Check sheet for the drawn part. Datum: minimum x, y, z corner. Units: mm. Give positions to 0.01 mm unless a question says otherwise; leave off trailing zeros. Write each loop counter-clockwise with the first axis right and the second up, starting at its lowest first coordinate (ties: lowest second). Pieces come first, ordered by that corner, then holes. Notation, with made-up numbers: (80, 10.25) -> (111, 10.25) arc R22 cw to (111, 40.25) -> close; hole circle Ø10 at (3.25, 41.25). An arc over 180 degrees is marked (long way). Write item = value, one per line. Start each with the question number.
1. Depth check by flat-ended pin: P1, Ø1.5, axis at x = 30, z = 3, coming from the -Y side; P2, Ø2, axis at y = 32.5, z = 3, coming from the +X side; P3, Ø0.7, axis at x = 29.5, z = 3, coming from the +Y side; P4, Ø5, axis at x = 24, y = 18.5, coming from the -Z side. Enter the tip coordinate at first touch or a pass-through.
2. Cross-section at D-D, the plane x = 26. Record the cut outline in (y, z).
3. Thickness scan on line 1 along Y through (x, z) = (16, 3.2); line 2 along Z through (x, y) = (30, 46); line 3 along X through (y, z) = (10, 5). Record the ranges inside material, lowest first.
4. Cross-section at A-A, the plane x = 16. Record the cut outline in (y, z).
5. Cross-section at B-B, the plane y = 11. Record the cut outline in (x, z), plus the area to 3 significant figures.
6. Mould release check, pull along Y, two halves, no side actions. Record for the marked faces 1, 2 and 3: pulls with the +Y half, pulls with the -Y half, needs draft (parallel to the pull), parting line crosses it, or undercut.
7. Cross-section at C-C, the plane x = 8. Record the cut outline in (y, z).
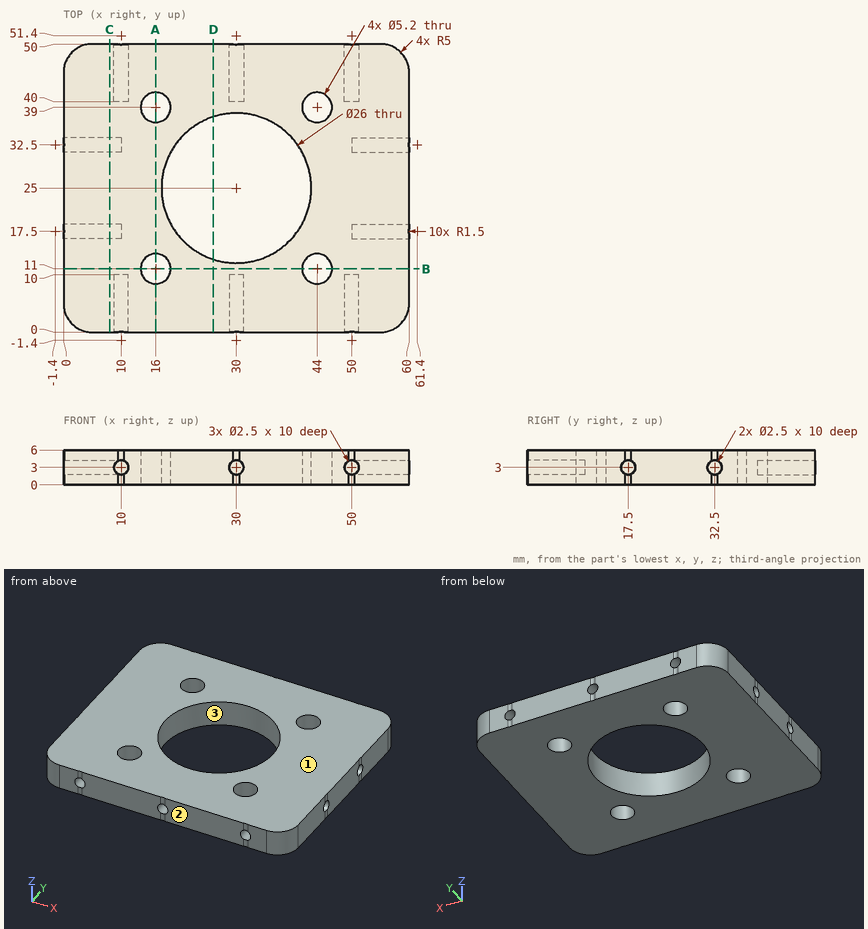
Answers:
q1.P1 = 10
q1.P2 = 50
q1.P3 = 40
q1.P4 = through
q2.outline = (0, 0) -> (12.63, 0) -> (12.63, 6) -> (0, 6) -> close; (37.37, 0) -> (50, 0) -> (50, 6) -> (37.37, 6) -> close
q3.line_1 = 0 to 8.4, 13.6 to 36.4, 41.6 to 50
q3.line_2 = 0 to 1.75, 4.25 to 6
q3.line_3 = 0 to 13.6, 18.4 to 41.6, 46.4 to 60
q4.outline = (0, 0) -> (8.4, 0) -> (8.4, 6) -> (0, 6) -> close; (13.6, 0) -> (36.4, 0) -> (36.4, 6) -> (13.6, 6) -> close; (41.6, 0) -> (50, 0) -> (50, 6) -> (41.6, 6) -> close
q5.outline = (0, 0) -> (13.4, 0) -> (13.4, 6) -> (0, 6) -> close; (18.6, 0) -> (41.4, 0) -> (41.4, 6) -> (18.6, 6) -> close; (46.6, 0) -> (60, 0) -> (60, 6) -> (46.6, 6) -> close
q5.area = 298 mm^2
q6.face_1 = needs draft
q6.face_2 = pulls with the -Y half
q6.face_3 = undercut
q7.outline = (0, 0) -> (50, 0) -> (50, 6) -> (0, 6) -> close; hole circle Ø2.5 at (17.5, 3); hole circle Ø2.5 at (32.5, 3)
